Work out the finished part from the listing and answer in its coordinate system (mm). A direction names the side the tool comes from. Coordinates: 2 decimals unless noted, no trailing zeros. Order: outer loops, then holes, each group sorted by start corner. A loop starts at its lowest first (then second) coordinate and runs counter-clockwise, first axis right, second up. Notation, with made-up numbers: M 8,-7.75 L 39,-7.75 A16 cw 39,-0.75 Z; hole C 64.5,1 d5. An arc over 180 degrees is marked long. Use a Markdown table: item, result. Add a question column.
from build123d import *

# Parameters (mm, degrees)
SZKIC1_W                    = 24
SZKIC1_H                    = 34
DODANIE_WYCI_GNI_CIE1_DEPTH = 1.4
SZKIC2_W                    = 20
SZKIC2_H                    = 30
SZKIC2_W_2                  = 16
SZKIC2_H_2                  = 26
DODANIE_WYCI_GNI_CIE2_DEPTH = 4
SZKIC3_W                    = 6.5
SZKIC3_H                    = 11
WYTNIJ_WYCI_GNI_CIE1_DEPTH  = 22.1896201
SZKIC4_W                    = 18
SZKIC4_H                    = 3
WYTNIJ_WYCI_GNI_CIE2_DEPTH  = 2
SZKIC5_W                    = 11
SZKIC5_H                    = 2.5
WYTNIJ_WYCI_GNI_CIE3_DEPTH  = 2
SFAZOWANIE1_SIZE            = 1.5
SFAZOWANIE1_SIZE_2          = 6
DODANIE_WYCI_GNI_CIE3_DEPTH = 1


with BuildPart() as part:
    # Szkic1 → Dodanie-wyciągnięcie1 (new body)
    with BuildSketch(Plane(origin=(0, 0, 0), x_dir=(1, 0, 0), z_dir=(0, 1, 0))):
        Rectangle(SZKIC1_W, SZKIC1_H)
    extrude(amount=DODANIE_WYCI_GNI_CIE1_DEPTH)

    # Szkic2 → Dodanie-wyciągnięcie2 (add)
    with BuildSketch(Plane.XZ):
        Rectangle(SZKIC2_W, SZKIC2_H)
        Rectangle(SZKIC2_W_2, SZKIC2_H_2, mode=Mode.SUBTRACT)
    extrude(amount=DODANIE_WYCI_GNI_CIE2_DEPTH)

    # Szkic3 → Wytnij-wyciągnięcie1 (cut, through all)
    with BuildSketch(Plane.XZ):
        with Locations((-4.75, -7.5)):
            Rectangle(SZKIC3_W, SZKIC3_H)
    extrude(amount=-WYTNIJ_WYCI_GNI_CIE1_DEPTH, mode=Mode.SUBTRACT)

    # Szkic4 → Wytnij-wyciągnięcie2 (cut)
    with BuildSketch(Plane.XY.offset(15)):
        with Locations((0, -2.5)):
            Rectangle(SZKIC4_W, SZKIC4_H)
    extrude(amount=-WYTNIJ_WYCI_GNI_CIE2_DEPTH, mode=Mode.SUBTRACT)

    # Szkic5 → Wytnij-wyciągnięcie3 (cut)
    with BuildSketch(Plane.ZY.offset(10)):
        with Locations((-7.5, -2.75)):
            Rectangle(SZKIC5_W, SZKIC5_H)
    extrude(amount=-WYTNIJ_WYCI_GNI_CIE3_DEPTH, mode=Mode.SUBTRACT)

    # Sfazowanie1
    # the kernel refuses this chamfer: 6, 1.5 mm, written as the material it takes off along each edge
    with BuildSketch(Plane(origin=(-8, -1.5, -13), x_dir=(-0.9890197255468893, -0.14778356633657133, 0), z_dir=(0, 0, 1))) as sfazowanie1_piece_1:
        Polygon((SFAZOWANIE1_SIZE * 0.989019725547, -SFAZOWANIE1_SIZE * 0.147783566337), (-SFAZOWANIE1_SIZE_2 * 0.147783566337, -SFAZOWANIE1_SIZE_2 * 0.989019725547), (0, 0), align=None)
    extrude(amount=11, mode=Mode.SUBTRACT)

    # Szkic6 → Dodanie-wyciągnięcie3 (add)
    with BuildSketch(Plane.XZ.offset(4)):
        Polygon((10, -15), (8, -15), (8, 13), (9, 13), (9, 15), (10, 15), (10, 13), align=None)
    extrude(amount=DODANIE_WYCI_GNI_CIE3_DEPTH)


solid = part.part
(1) The mould has two halves that part along X. Classify faces 1 (the flat face through (0, -0.6, 15)), 2 (the flat face through (12, 1, 0)), 3 (the flat face through (8, -2, -1)), 4 (the flat face through (-12, 1, 0)): pulls with the +X half, pulls with the -X half, needs draft (parallel to the pull), parting line crosses it, or undercut.
(2) A cutting plane is placed at D-D on x = 4. Write down the section's boundary in (y, z), plus the area to 3 significant figures.
(3) Straight lines are drawn through the part: line 1 (X direction, y = -1.5, z = 6.5); line 2 (Z direction, x = -6, y = 0.5); line 3 (Z direction, x = -7, y = -0.5). For each, find the intervals that lie inside material, in ascending order.
(4) Given P1, Ø1.5, axis at y = -3, z = 0.5, coming from the -X side; P2, Ø0.6, axis at x = -4, z = -14, coming from the -Y side; P3, Ø2, axis at y = -1.5, z = 10.5, coming from the +X side; P4, Ø10, axis at x = -7.5, z = -9.5, coming from the +Y side, each flat-ended and moving along its own axis, determine where each tip first touches the part or whether it passes through.
(5) A cutting plane is placed at C-C on y = -0.5. Write down the section's boundary in (x, z).
(6) A cutting plane is placed at B-B on y = -3. Write down the section's boundary in (x, z), plus the area to 3 significant figures.
(7) Which of the six approach directions +Z, -Z, +X, -X, +Y, -Y give full straight-line access (tool end or side, diameter ignored) to faces 5 (the flat face through (0, -2, -15)), 6 (the flat face through (-1, -4, -14)), 7 (the flat face through (-6.7, 0.2, -2)), 8 (the flat face through (0, -1, 14))?
(8) A cutting plane is placed at A-A on z = -6.5. Write down the section's boundary in (x, y) (3 decimals).
From the geometry:
| question | item | result |
|---|---|---|
| 1 | face 1 | needs draft |
| 1 | face 2 | pulls with the +X half |
| 1 | face 3 | undercut |
| 1 | face 4 | pulls with the -X half |
| 2 | outline | M -4,-15 L 0,-15 L 0,-17 L 1.4,-17 L 1.4,17 L 0,17 L 0,15 L -1,15 L -1,13 L 0,13 L 0,-13 L -4,-13 Z |
| 2 | area | 57.6 mm2 |
| 3 | line 1 | x = -10 to -8, 8 to 10 |
| 3 | line 2 | z = -17 to -13, -2 to 17 |
| 3 | line 3 | z = -15 to -13, 13 to 15 |
| 4 | P1 | stops at x = -10 |
| 4 | P2 | stops at y = -4 |
| 4 | P3 | stops at x = 10 |
| 4 | P4 | stops at y = 1.4 |
| 5 | outline | M -10,-15 L 10,-15 L 10,15 L -10,15 Z; hole M -9.25,-13 L 8,-13 L 8,13 L -8,13 L -8,-2 L -9.25,-2 Z |
| 6 | outline | M -10,-15 L 10,-15 L 10,15 L 9,15 L 9,13 L 8,13 L 8,-13 L -10,-13 Z; M -10,-2 L -8,-2 L -8,13 L -9,13 L -9,15 L -10,15 Z |
| 6 | area | 126 mm2 |
| 7 | face 5 | -Z, +X, -X, -Y |
| 7 | face 6 | +Z, -Z, -X, -Y |
| 7 | face 7 | -Y |
| 7 | face 8 | +Z, -Y |
| 8 | outline | M -12,0 L -10,0 L -10,-1.5 L -9.5,-1.5 L -8.775,1.4 L -12,1.4 Z; M -1.5,0 L 8,0 L 8,-5 L 10,-5 L 10,0 L 12,0 L 12,1.4 L -1.5,1.4 Z |
